Check sheet for the modelled part. Datum: model origin and axes. Units: mm. Face numbers are marked on the shaded views. A direction names the side the tool comes from. Give positions to 0.01 mm unless a question says otherwise; leave off trailing zeros. Write each loop counter-clockwise with the first axis right and the second up, starting at its lowest first coordinate (ties: lowest second). Pieces come first, ordered by that corner, then holes. Notation, with made-up numbers: M -7,-19 L 39,-19 A36 cw 39,15 Z; hole C 0,24 d6. An arc over 180 degrees is marked long. Write item = value, one per line. Start each with the question number.
1) Access from +Z, -Z, +X, -X, +Y, -Y to the whole of each face (thin tool, end or side, straight path). Record for the marked faces 1, 2, 3, 4 and 5.
2) Cross-section at D-D, the plane y = 3.75. Record the cut outline in (x, z), plus the area to 3 significant figures.
3) Cross-section at B-B, the plane y = 16.25. Record the cut outline in (x, z), plus the area to 3 significant figures.
4) Go/stop test with flat-tipped pins: pin 1 (5 mm diameter, centred on x = 9.5, y = 10, fed in from -Z); pin 2 (1.8 mm diameter, centred on x = 13, y = 13.5, fed in from +Z); pin 3 (1.5 mm diameter, centred on x = 9, y = 59.5, fed in from +Z). Record where each tip stops, or that it passes through.
5) Cross-section at A-A, the plane x = 14. Record the cut outline in (y, z), plus the area to 3 significant figures.
6) Cross-section at C-C, the plane x = 10. Record the cut outline in (y, z), plus the area to 3 significant figures.
7) Scan lines: line 1 along Y through (x, z) = (14, 2.05); line 2 along X through (y, z) = (23, 25); line 3 along Z through (x, y) = (14, 8). Record each from-to range of solid material in increasing order. Write a range as [from, to].
```python
from build123d import *

# Parameters (mm, degrees)
SKETCH_1_W          = 17
SKETCH_1_H          = 20
SKETCH_1_R          = 1.5
EXTRUDE_1_DEPTH     = 3
EXTRUDE_2_DEPTH     = 5
SKETCH_4_R          = 1.5
CUT_EXTRUDE_1_DEPTH = 5
FILLET_2_R          = 5
FILLET_3_R          = 1.3
FILLET_4_R          = 10
SKETCH_5_W          = 6
SKETCH_5_H          = 20
CUT_EXTRUDE_2_DEPTH = 10
SKETCH_6_R          = 1.5
CUT_EXTRUDE_3_DEPTH = 1


with BuildPart() as part:
    # 草图1 → 凸台-拉伸1 (new body)
    with BuildSketch(Plane.XY):
        with Locations((8.5, 10)):
            Rectangle(SKETCH_1_W, SKETCH_1_H)
        with Locations((3, 16.25)):
            Circle(SKETCH_1_R, mode=Mode.SUBTRACT)
        with Locations((14, 16.25)):
            Circle(SKETCH_1_R, mode=Mode.SUBTRACT)
        with Locations((14, 3.75)):
            Circle(SKETCH_1_R, mode=Mode.SUBTRACT)
        with Locations((3, 3.75)):
            Circle(SKETCH_1_R, mode=Mode.SUBTRACT)
    extrude(amount=EXTRUDE_1_DEPTH)

    # 草图3 → 凸台-拉伸2 (add)
    with BuildSketch(Plane.ZY.offset(-6)):
        Polygon((3, 20), (5.309401077, 20), (-16.607695155, 57.961524227), (0.712812921, 67.961524227), (30.712812921, 16), (3, 0), align=None)
    extrude(amount=-EXTRUDE_2_DEPTH)

    # 草图4 → 切除-拉伸1 (cut)
    with BuildSketch(Plane(origin=(11, 0, 0), x_dir=(0, 0, -1), z_dir=(1, 0, 0))):
        with Locations((-5.898711306, 50.979284742)):
            Circle(SKETCH_4_R)
        with Locations((10.493593539, 55.371589587)):
            Circle(SKETCH_4_R)
    extrude(amount=-CUT_EXTRUDE_1_DEPTH, mode=Mode.SUBTRACT)

    # 圆角2
    fillet_2_edges = [part.edges().sort_by_distance(p)[0] for p in [
        (8.5, 57.961524227, -16.607695155),
        (8.5, 67.961524227, 0.712812921),
    ]]
    fillet(fillet_2_edges, radius=FILLET_2_R)

    # 圆角3
    fillet_3_edges = [part.edges().sort_by_distance(p)[0] for p in [
        (8.5, 20, 5.309401077),
    ]]
    fillet(fillet_3_edges, radius=FILLET_3_R)

    # 圆角4
    fillet_4_edges = [part.edges().sort_by_distance(p)[0] for p in [
        (8.5, 16, 30.712812921),
    ]]
    fillet(fillet_4_edges, radius=FILLET_4_R)

    # 草图5 → 切除-拉伸2 (cut)
    with BuildSketch(Plane.XY.offset(3)):
        with Locations((3, 10)):
            Rectangle(SKETCH_5_W, SKETCH_5_H)
    extrude(amount=-CUT_EXTRUDE_2_DEPTH, mode=Mode.SUBTRACT)

    # 草图6 → 切除-拉伸3 (cut)
    with BuildSketch(Plane.ZY.offset(-6)):
        with BuildLine():
            Line((3, 0), (22.052558883, 11))
            ThreePointArc((22.052558883, 11), (26.711817146, 17.072063587), (25.712812921, 24.660254038))
            Line((25.712812921, 24.660254038), (3.212812921, 63.631397208))
            ThreePointArc((3.212812921, 63.631397208), (0.176781128, 65.96102634), (-3.617314098, 65.461524227))
            Line((-3.617314098, 65.461524227), (-12.277568136, 60.461524227))
            ThreePointArc((-12.277568136, 60.461524227), (-14.607197267, 57.425492434), (-14.107695155, 53.631397208))
            Line((-14.107695155, 53.631397208), (4.183568052, 21.95))
            ThreePointArc((4.183568052, 21.95), (4.183568052, 20.65), (3.057735027, 20))
            Line((3.057735027, 20), (0, 20))
            Line((0, 20), (0, 0))
            Line((0, 0), (3, 0))
        make_face()
        with Locations((5.898711306, 50.979284742)):
            Circle(SKETCH_6_R, mode=Mode.SUBTRACT)
        with Locations((-10.493593539, 55.371589587)):
            Circle(SKETCH_6_R, mode=Mode.SUBTRACT)
    extrude(amount=-CUT_EXTRUDE_3_DEPTH, mode=Mode.SUBTRACT)


solid = part.part
```
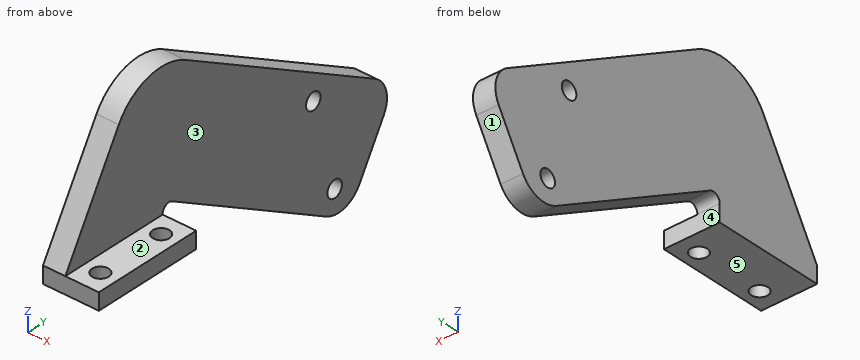
Reply:
q1.face_1 = -Z, +X, -X, +Y
q1.face_2 = +Z, +X, +Y, -Y
q1.face_3 = +Z, +X, +Y
q1.face_4 = -Z, +X, -X
q1.face_5 = -Z, +X, -X, -Y
q2.outline = M 7,0 L 12.5,0 L 12.5,3 L 11,3 L 11,9.5 L 7,9.5 Z; M 15.5,0 L 17,0 L 17,3 L 15.5,3 Z
q2.area = 47.0 mm2
q3.outline = M 7,0 L 12.5,0 L 12.5,3 L 11,3 L 11,26.45 L 7,26.45 Z; M 15.5,0 L 17,0 L 17,3 L 15.5,3 Z
q3.area = 115 mm2
q4.pin_1 = 0
q4.pin_2 = 3
q4.pin_3 = 6.03
q5.outline = M 0,0 L 2.25,0 L 2.25,3 L 0,3 Z; M 5.25,0 L 14.75,0 L 14.75,3 L 5.25,3 Z; M 17.75,0 L 20,0 L 20,3 L 17.75,3 Z
q5.area = 42.0 mm2
q6.outline = M 0,0 L 20,0 L 20,3.06 A1.3 cw 21.95,4.18 L 53.63,-14.11 A5 ccw 60.46,-12.28 L 65.46,-3.62 A5 ccw 63.63,3.21 L 24.66,25.71 A10 ccw 11,22.05 L 0,3 Z; hole C 50.98,5.9 d3; hole C 55.37,-10.49 d3
q6.area = 1,330 mm2
q7.line_1 = [0, 2.25], [5.25, 14.75], [17.75, 20]
q7.line_2 = [7, 11]
q7.line_3 = [0, 3]
